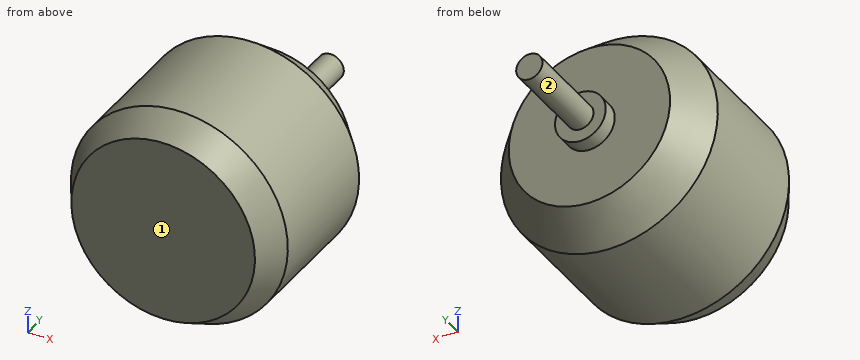
from build123d import *

# Parameters (mm, degrees)
SKETCH2_R           = 3
BOSS_EXTRUDE1_DEPTH = 24.39
SKETCH4_R           = 5.79
BOSS_EXTRUDE2_DEPTH = 3.66


with BuildPart() as part:
    # Sketch1 → Revolve1 (revolve)
    with BuildSketch(Plane.XY, mode=Mode.PRIVATE) as revolve1_sk:
        Polygon((0, 0), (0, 43.64), (18.418686804, 43.64), (24.76, 35.523489238), (24.76, 6.581793069), (20.96, 0), align=None)
    revolve(revolve1_sk.sketch.rotate(Axis((0, 0, 0), (0, 1, 0)), 90), axis=Axis((0, 0, 0), (0, 1, 0)))

    # Sketch2 → Boss-Extrude1 (add)
    with BuildSketch(Plane(origin=(0, 43.64, 0), x_dir=(1, 0, 0), z_dir=(0, 1, 0))):
        with Locations(Location((0, 0, 0), (0, 0, 270))):
            Circle(SKETCH2_R)
    extrude(amount=BOSS_EXTRUDE1_DEPTH)

    # Sketch4 → Boss-Extrude2 (add)
    with BuildSketch(Plane(origin=(0, 43.64, 0), x_dir=(1, 0, 0), z_dir=(0, 1, 0))):
        with Locations(Location((0, 0, 0), (0, 0, 270))):
            Circle(SKETCH4_R)
    extrude(amount=BOSS_EXTRUDE2_DEPTH)


solid = part.part
Could you check a few things on this model? Use its own coordinates, in mm. Face numbers are marked on the shaded views. A direction names the side the tool comes from. Round coordinates to 2 decimals unless told otherwise and drop trailing zeros. Loops run counter-clockwise (first coordinate to the right, second up) from the corner with the lowest first, then second, coordinate; pieces in that order, holes last. Notation, with made-up numbers: (48, 73) -> (107, 73) arc R19 cw to (107, 107) -> close; hole circle Ø4 at (40, -33). An arc over 180 degrees is marked (long way). Use CSV: the item, a comma, the result in double quotes.
(1) Suppose I cut it at D-D on y = 42. Write out the boundary of the cut face in (x, z).
Return value:
outline,"circle Ø39.4 at (0, 0)"
(2) Suppose I cut it at A-A on x = 0. Write out the boundary of the cut face in (y, z), plus the area to 3 significant figures.
Return value:
outline,"(0, -20.96) -> (6.58, -24.76) -> (35.52, -24.76) -> (43.64, -18.42) -> (43.64, -5.79) -> (47.3, -5.79) -> (47.3, -3) -> (68.03, -3) -> (68.03, 3) -> (47.3, 3) -> (47.3, 5.79) -> (43.64, 5.79) -> (43.64, 18.42) -> (35.52, 24.76) -> (6.58, 24.76) -> (0, 20.96) -> close"
area,"2,250 mm²"
(3) For the marked faces 1 and 2, which set-ups out of +Z, -Z, +X, -X, +Y, -Y let a thin tool reach every point of the face, with its end or its side?
Return value:
face 1,"+Z, -Z, +X, -X, -Y"
face 2,"+Y"
(4) Will these pins go through, and if not, where does the flat tip stop? pin 1 Ø3 at (x, z) = (-6, 16.5) entering from +Y; pin 2 Ø2 at (x, y) = (4, 19.5) entering from -Z; pin 3 Ø8 at (y, z) = (31, 10.5) entering from -X.
Return value:
pin 1,"stops at y = 43.64"
pin 2,"stops at z = -24.58"
pin 3,"stops at x = -23.89"
(5) Suppose I cut it at B-B on z = 0. Write out the boundary of the cut face in (x, y).
Return value:
outline,"(-24.76, 6.58) -> (-20.96, 0) -> (20.96, 0) -> (24.76, 6.58) -> (24.76, 35.52) -> (18.42, 43.64) -> (5.79, 43.64) -> (5.79, 47.3) -> (3, 47.3) -> (3, 68.03) -> (-3, 68.03) -> (-3, 47.3) -> (-5.79, 47.3) -> (-5.79, 43.64) -> (-18.42, 43.64) -> (-24.76, 35.52) -> close"
(6) If I drill on probe 1 along Y at (x, z) = (-3, 15.5); probe 2 along Y at (x, z) = (-3.5, -1); probe 3 along X at (y, z) = (12, 4), over which ranges is the centre line in solid material (lowest first)? Write a range as [from, to].
Return value:
probe 1,"y = [0, 43.64]"
probe 2,"y = [0, 47.3]"
probe 3,"x = [-24.43, 24.43]"
(7) Suppose I cut it at C-C on y = 56. Write out the boundary of the cut face in (x, z), plus the area to 3 significant figures.
Return value:
outline,"circle Ø6 at (0, 0)"
area,"28.3 mm²"
